Source: CAD feature listing. Evaluate the final solid. Frame: model axes, mm. A direction names the side the tool comes from. Give positions to 0.01 mm unless a question says otherwise; leave off trailing zeros. Write each loop counter-clockwise with the first axis right and the second up, starting at its lowest first coordinate (ties: lowest second). Pieces come first, ordered by that corner, then holes. Notation, with made-up numbers: M 85,1.5 L 91,1.5 A22 cw 91,35.5 Z; hole C -21,28 d9. An arc over 180 degrees is marked long. Answer as a JSON object with one key per item and string values. Group by question number.
```python
from build123d import *

# Parameters (mm, degrees)
SKETCH1_R           = 12
BOSS_EXTRUDE1_DEPTH = 50
SKETCH2_R           = 13
BOSS_EXTRUDE2_DEPTH = 2
SKETCH3_R           = 55
BOSS_EXTRUDE3_DEPTH = 3
BOSS_EXTRUDE4_DEPTH = 131
BOSS_EXTRUDE5_DEPTH = 39
SKETCH6_R           = 4.5
CUT_EXTRUDE1_DEPTH  = 15
SKETCH7_W           = 41
SKETCH7_H           = 41
BOSS_EXTRUDE6_DEPTH = 46


with BuildPart() as part:
    # Sketch1 → Boss-Extrude1 (new body)
    with BuildSketch(Plane.XY):
        Circle(SKETCH1_R)
    extrude(amount=-BOSS_EXTRUDE1_DEPTH)

    # Sketch2 → Boss-Extrude2 (add)
    with BuildSketch(Plane(origin=(0, 0, -50), x_dir=(-1, 0, 0), z_dir=(0, 0, -1))):
        Circle(SKETCH2_R)
    extrude(amount=BOSS_EXTRUDE2_DEPTH)

    # Sketch3 → Boss-Extrude3 (add)
    with BuildSketch(Plane(origin=(0, 0, -52), x_dir=(-1, 0, 0), z_dir=(0, 0, -1))):
        Circle(SKETCH3_R)
    extrude(amount=BOSS_EXTRUDE3_DEPTH)

    # Sketch4 → Boss-Extrude4 (add)
    with BuildSketch(Plane(origin=(0, 0, -55), x_dir=(-1, 0, 0), z_dir=(0, 0, -1))):
        with BuildLine():
            Line((-50.806003582, -65), (50.806003582, -65))
            ThreePointArc((50.806003582, -65), (58.336309448, -58.336309448), (65, -50.806003582))
            Line((65, -50.806003582), (65, 50.806003582))
            ThreePointArc((65, 50.806003582), (58.336309448, 58.336309448), (50.806003582, 65))
            Line((50.806003582, 65), (-50.806003582, 65))
            ThreePointArc((-50.806003582, 65), (-58.336309448, 58.336309448), (-65, 50.806003582))
            Line((-65, 50.806003582), (-65, -50.806003582))
            ThreePointArc((-65, -50.806003582), (-58.336309448, -58.336309448), (-50.806003582, -65))
        make_face()
    extrude(amount=BOSS_EXTRUDE4_DEPTH)

    # Sketch5 → Boss-Extrude5 (add)
    with BuildSketch(Plane(origin=(0, 0, -186), x_dir=(-1, 0, 0), z_dir=(0, 0, -1))):
        with BuildLine():
            Line((-19.5, -34.92491947), (-19.5, -81.5))
            Line((-19.5, -81.5), (19.5, -81.5))
            Line((19.5, -81.5), (19.5, -34.92491947))
            ThreePointArc((19.5, -34.92491947), (0, 40), (-19.5, -34.92491947))
        make_face()
    extrude(amount=BOSS_EXTRUDE5_DEPTH)

    # Sketch6 → Cut-Extrude1 (cut)
    with BuildSketch(Plane.XY.offset(-55)):
        with Locations((-51.265241636, 51.265241636)):
            Circle(SKETCH6_R)
        with Locations((51.265241636, 51.265241636)):
            Circle(SKETCH6_R)
        with Locations((51.265241636, -51.265241636)):
            Circle(SKETCH6_R)
        with Locations((-51.265241636, -51.265241636)):
            Circle(SKETCH6_R)
    extrude(amount=-CUT_EXTRUDE1_DEPTH, mode=Mode.SUBTRACT)

    # Sketch7 → Boss-Extrude6 (add)
    with BuildSketch(Plane.XZ.offset(65)):
        with Locations((0, -156.5)):
            Rectangle(SKETCH7_W, SKETCH7_H)
    extrude(amount=BOSS_EXTRUDE6_DEPTH)


solid = part.part
```
(1) Section D-D, the plane z = -60.5. Return loops of the section in (x, y).
(2) Pull-direction query (Z, two-part tool) for faces 5 (the flat face through (0, -88, -177)), 6 (the flat face through (-51, 51, -70)), 7 (the flat face through (65, 1, -120)); classes: pulls with the +Z half, pulls with the -Z half, needs draft (parallel to the pull), parting line crosses it, or undercut.
(3) Ray query, L1, parallel to X at y = -40, z = -189; L2, parallel to Y at x = -44.5, z = -168.5; L3, parallel to Z at x = 36, y = -37.5. Return the intervals inside material, ascending. Write a range as [from, to].
(4) Contact query for flat-ended pins moving along their axis: pin 1 Ø11.5 at (x, z) = (-1.5, -206) entering from -Y; pin 2 Ø1 at (y, z) = (-60.5, -97.5) entering from +X; pin 3 Ø6 at (x, z) = (3.5, -134.5) entering from -Y; pin 4 Ø18 at (x, y) = (6, -74.5) entering from +Z. Output: stop coordinate, or through.
(5) Section A-A, the plane x = 0. Return loops of the section in (y, z).
(6) Section B-B, the plane z = -109. Return loops of the section in (x, y).
(7) Access query for faces 1 (the cylindrical face through (-1.474, 39.973, -205.227)), 2 (the flat face through (-20.5, -88, -157)), 3 (the cylindrical face through (11.923, -53.692, -53.479)), 4 (the flat face through (20.5, -88, -157)). Directions: +Z, -Z, +X, -X, +Y, -Y. A direction counts if a zero-diameter tool reaches every point of the face in a straight line with its end or side. Return the directions, or none.
(8) Section C-C, the plane y = 0. Return loops of the section in (x, z), plus the area to 3 significant figures.
Reported:
{
 "1": {"outline": "M -65,-50.81 A82.5 ccw -50.81,-65 L 50.81,-65 A82.5 ccw 65,-50.81 L 65,50.81 A82.5 ccw 50.81,65 L -50.81,65 A82.5 ccw -65,50.81 Z; hole C -51.27,-51.27 d9; hole C -51.27,51.27 d9; hole C 51.27,-51.27 d9; hole C 51.27,51.27 d9"},
 "2": {"face 5": "undercut", "face 6": "pulls with the +Z half", "face 7": "needs draft"},
 "3": {"L1": "x = [-19.5, 19.5]", "L2": "y = [-65, 65]", "L3": "z = [-186, -52]"},
 "4": {"pin 1": "stops at y = -81.5", "pin 2": "stops at x = 56.62", "pin 3": "stops at y = -111", "pin 4": "stops at z = -136"},
 "5": {"outline": "M -111,-177 L -65,-177 L -65,-186 L -81.5,-186 L -81.5,-225 L 40,-225 L 40,-186 L 65,-186 L 65,-55 L 55,-55 L 55,-52 L 13,-52 L 13,-50 L 12,-50 L 12,0 L -12,0 L -12,-50 L -13,-50 L -13,-52 L -55,-52 L -55,-55 L -65,-55 L -65,-136 L -111,-136 Z"},
 "6": {"outline": "M -65,-50.81 A82.5 ccw -50.81,-65 L 50.81,-65 A82.5 ccw 65,-50.81 L 65,50.81 A82.5 ccw 50.81,65 L -50.81,65 A82.5 ccw -65,50.81 Z"},
 "7": {"face 1": "-Z", "face 2": "+Z, -Z, -X, -Y", "face 3": "+Z", "face 4": "+Z, -Z, +X, -Y"},
 "8": {"outline": "M -65,-186 L -40,-186 L -40,-225 L 40,-225 L 40,-186 L 65,-186 L 65,-55 L 55,-55 L 55,-52 L 13,-52 L 13,-50 L 12,-50 L 12,0 L -12,0 L -12,-50 L -13,-50 L -13,-52 L -55,-52 L -55,-55 L -65,-55 Z", "area": "21,700 mm2"}
}
